Could you check a few things on this model? Use its own coordinates, in mm. Give positions to 0.01 mm unless a question says otherwise; leave off trailing zeros. Write each loop counter-clockwise with the first axis right and the second up, starting at its lowest first coordinate (ties: lowest second). Pieces come first, ordered by that corner, then holes. Notation, with made-up numbers: M -19.5,55.25 L 26.5,55.25 A24 cw 26.5,93.25 Z; hole C -34.75,14 d3. An arc over 180 degrees is marked long. One line per item, written item: value.
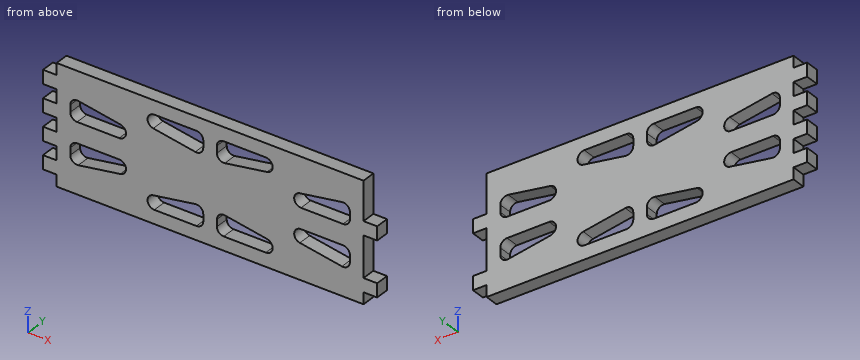
```python
from build123d import *

# Parameters (mm, degrees)
BOSS_EXTRUDE1_DEPTH = 4
CUT_EXTRUDE1_DEPTH  = 10


with BuildPart() as part:
    # Sketch1 → Boss-Extrude1 (new body)
    with BuildSketch(Plane(origin=(0, 0, 0), x_dir=(1, 0, 0), z_dir=(0, 1, 0))):
        Polygon((-13.523809524, 16), (-17.523809524, 16), (-17.523809524, 12), (-13.523809524, 12), (-13.523809524, 8), (-17.523809524, 8), (-17.523809524, 4), (-13.523809524, 4), (-13.523809524, 0), (-17.523809524, 0), (-17.523809524, -4), (-13.523809524, -4), (-13.523809524, -8), (-17.523809524, -8), (-17.523809524, -12), (-13.523809524, -12), (-13.523809524, -15.38), (76.476190476, -15.38), (76.476190476, -4), (80.476190476, -4), (80.476190476, 0), (76.476190476, 0), (76.476190476, 12), (80.476190476, 12), (80.476190476, 16), (76.476190476, 16), (76.476190476, 19.38), (-13.523809524, 19.38), align=None)
    extrude(amount=-BOSS_EXTRUDE1_DEPTH)

    # Sketch2 → Cut-Extrude1 (cut)
    with BuildSketch(Plane(origin=(0, 0, 0), x_dir=(1, 0, 0), z_dir=(0, 1, 0))):
        with BuildLine():
            ThreePointArc((-9.523809524, 9.071498058), (-8.815677287, 10.598284776), (-7.192731841, 11.0439046))
            Line((-7.192731841, 11.0439046), (5.148288204, 8.972406542))
            ThreePointArc((5.148288204, 8.972406542), (6.810300218, 6.833887214), (4.817210521, 5))
            Line((4.817210521, 5), (-7.523809524, 5))
            ThreePointArc((-7.523809524, 5), (-8.938023086, 5.585786438), (-9.523809524, 7))
            Line((-9.523809524, 7), (-9.523809524, 9.071498058))
        make_face()
        with BuildLine():
            Line((15.135170432, 15.38), (27.476190476, 15.38))
            ThreePointArc((27.476190476, 15.38), (28.890404039, 14.794213562), (29.476190476, 13.38))
            Line((29.476190476, 13.38), (29.476190476, 11.308501942))
            ThreePointArc((29.476190476, 11.308501942), (28.768058239, 9.781715224), (27.145112793, 9.3360954))
            Line((27.145112793, 9.3360954), (14.804092749, 11.407593458))
            ThreePointArc((14.804092749, 11.407593458), (13.142080734, 13.546112786), (15.135170432, 15.38))
        make_face()
        with BuildLine():
            Line((33.476190476, 13.38), (33.476190476, 11.308501942))
            ThreePointArc((33.476190476, 11.308501942), (34.184322713, 9.781715224), (35.807268159, 9.3360954))
            Line((35.807268159, 9.3360954), (48.148288204, 11.407593458))
            ThreePointArc((48.148288204, 11.407593458), (49.810300218, 13.546112786), (47.817210521, 15.38))
            Line((47.817210521, 15.38), (35.476190476, 15.38))
            ThreePointArc((35.476190476, 15.38), (34.061976914, 14.794213562), (33.476190476, 13.38))
        make_face()
        with BuildLine():
            ThreePointArc((72.476190476, 7), (71.890404039, 5.585786438), (70.476190476, 5))
            Line((70.476190476, 5), (58.135170432, 5))
            ThreePointArc((58.135170432, 5), (56.142080734, 6.833887214), (57.804092749, 8.972406542))
            Line((57.804092749, 8.972406542), (70.145112793, 11.0439046))
            ThreePointArc((70.145112793, 11.0439046), (71.768058239, 10.598284776), (72.476190476, 9.071498058))
            Line((72.476190476, 9.071498058), (72.476190476, 7))
        make_face()
        with BuildLine():
            ThreePointArc((72.476190476, -5.071498058), (71.768058239, -6.598284776), (70.145112793, -7.0439046))
            Line((70.145112793, -7.0439046), (57.804092749, -4.972406542))
            ThreePointArc((57.804092749, -4.972406542), (56.142080734, -2.833887214), (58.135170432, -1))
            Line((58.135170432, -1), (70.476190476, -1))
            ThreePointArc((70.476190476, -1), (71.890404039, -1.585786438), (72.476190476, -3))
            Line((72.476190476, -3), (72.476190476, -5.071498058))
        make_face()
        with BuildLine():
            Line((47.817210521, -11.38), (35.476190476, -11.38))
            ThreePointArc((35.476190476, -11.38), (34.061976914, -10.794213562), (33.476190476, -9.38))
            Line((33.476190476, -9.38), (33.476190476, -7.308501942))
            ThreePointArc((33.476190476, -7.308501942), (34.184322713, -5.781715224), (35.807268159, -5.3360954))
            Line((35.807268159, -5.3360954), (48.148288204, -7.407593458))
            ThreePointArc((48.148288204, -7.407593458), (49.810300218, -9.546112786), (47.817210521, -11.38))
        make_face()
        with BuildLine():
            Line((29.476190476, -9.38), (29.476190476, -7.308501942))
            ThreePointArc((29.476190476, -7.308501942), (28.768058239, -5.781715224), (27.145112793, -5.3360954))
            Line((27.145112793, -5.3360954), (14.804092749, -7.407593458))
            ThreePointArc((14.804092749, -7.407593458), (13.142080734, -9.546112786), (15.135170432, -11.38))
            Line((15.135170432, -11.38), (27.476190476, -11.38))
            ThreePointArc((27.476190476, -11.38), (28.890404039, -10.794213562), (29.476190476, -9.38))
        make_face()
        with BuildLine():
            ThreePointArc((-9.523809524, -3), (-8.938023086, -1.585786438), (-7.523809524, -1))
            Line((-7.523809524, -1), (4.817210521, -1))
            ThreePointArc((4.817210521, -1), (6.810300218, -2.833887214), (5.148288204, -4.972406542))
            Line((5.148288204, -4.972406542), (-7.192731841, -7.0439046))
            ThreePointArc((-7.192731841, -7.0439046), (-8.815677287, -6.598284776), (-9.523809524, -5.071498058))
            Line((-9.523809524, -5.071498058), (-9.523809524, -3))
        make_face()
    extrude(amount=-CUT_EXTRUDE1_DEPTH, mode=Mode.SUBTRACT)


solid = part.part
```
1) If we section it at C-C, the plane y = -0.8: Give the number of separate pieces and of enclosed holes in the cut face, then the cut area to 3 significant figures.
Outcome:
separate pieces: 1
enclosed holes: 8
area: 2,590 mm^2
2) I'm going to push flat-ended pins straight in: pin 1 (2 mm diameter, centred on x = -16, y = -2, fed in from +Z); pin 2 (2 mm diameter, centred on x = 78.5, y = -2.5, fed in from +Z); pin 3 (1.5 mm diameter, centred on x = 26.5, z = -13.5, fed in from -Y); pin 4 (0.6 mm diameter, centred on y = -2.5, z = 4.5, fed in from +X). Where does each tip first touch, or does it pass through?
Outcome:
pin 1: stops at z = 12
pin 2: stops at z = 4
pin 3: passes through
pin 4: stops at x = 76.48
3) If we section it at A-A, the plane x = -5.5: Write out the boundary of the cut face in (y, z), then the cut area to 3 significant figures.
Outcome:
outline: M -4,-19.38 L 0,-19.38 L 0,-10.76 L -4,-10.76 Z; M -4,-5 L 0,-5 L 0,1 L -4,1 Z; M -4,6.76 L 0,6.76 L 0,15.38 L -4,15.38 Z
area: 93.0 mm^2
4) Please list where these lines run through material, in increasing order: L1, parallel to X at y = -1.35, z = 3; L2, parallel to Z at x = 3, y = -1.85; L3, parallel to X at y = -2.5, z = 8.5. Write a range as from..to.
Outcome:
L1: x = -17.52..-9.52, 6.82..56.14, 72.48..80.48
L2: z = -19.38..-9.33, -5..1, 5.33..15.38
L3: x = -17.52..13.34, 29.48..33.48, 49.61..76.48
5) If we section it at B-B, the plane x = 40.5: Write out the boundary of the cut face in (y, z), then the cut area to 3 significant figures.
Outcome:
outline: M -4,-19.38 L 0,-19.38 L 0,-15.38 L -4,-15.38 Z; M -4,-10.12 L 0,-10.12 L 0,6.12 L -4,6.12 Z; M -4,11.38 L 0,11.38 L 0,15.38 L -4,15.38 Z
area: 97.0 mm^2
